```python
from build123d import *

# Parameters (mm, degrees)
EXTRUDE_1_DEPTH     = 30
CHAMFER_1_SIZE      = 5
SKETCH_2_R          = 4
CUT_EXTRUDE_2_DEPTH = 58.295890515
SKETCH_3_R          = 4
CUT_EXTRUDE_3_DEPTH = 61.952262634


with BuildPart() as part:
    # Эскиз1 → Вытянуть1 (new body)
    with BuildSketch(Plane.XY):
        Polygon((15, 7.896395833), (35, 7.896395833), (44.894389845, -8.278473804), (44.894389845, -28.278473804), (35, -28.278473804), (35, -8.278473804), (15, -8.278473804), (15, -28.278473804), (5.105610155, -28.278473804), (5.105610155, -8.278473804), align=None)
    extrude(amount=EXTRUDE_1_DEPTH)

    # Фаска1
    chamfer_1_edges = [part.edges().sort_by_distance(p)[0] for p in [
        (10.052805078, -28.278473804, 0),
        (39.947194922, -28.278473804, 0),
        (10.052805078, -28.278473804, 30),
        (39.947194922, -28.278473804, 30),
    ]]
    chamfer(chamfer_1_edges, length=CHAMFER_1_SIZE)

    # Эскиз2 → Вытянуть2 (cut, through all)
    with BuildSketch(Plane.ZY.offset(-5.105610155)):
        with Locations((15, -18.278473804)):
            Circle(SKETCH_2_R)
    extrude(amount=-CUT_EXTRUDE_2_DEPTH, mode=Mode.SUBTRACT)

    # Эскиз3 → Вытянуть3 (cut, through all)
    with BuildSketch(Plane.XY.offset(30)):
        with Locations((25, -0.278473804)):
            Circle(SKETCH_3_R)
    extrude(amount=-CUT_EXTRUDE_3_DEPTH, mode=Mode.SUBTRACT)


solid = part.part
```
Check sheet for the modelled part. Datum: model origin and axes. Units: mm. A direction names the side the tool comes from. Round coordinates to 2 decimals unless told otherwise and drop trailing zeros. Loops run counter-clockwise (first coordinate to the right, second up) from the corner with the lowest first, then second, coordinate; pieces in that order, holes last. Notation, with made-up numbers: M 56,75 L 106,75 A32 ccw 106,107 Z; hole C 4.25,-40 d9. An arc over 180 degrees is marked long. Answer as a JSON object with one key per item and string values.
1. Section check D-D (z = 21). Record the boundary of the cut face in (x, y), plus the area to 3 significant figures.
Reply:
{"outline": "M 5.11,-28.28 L 15,-28.28 L 15,-8.28 L 35,-8.28 L 35,-28.28 L 44.89,-28.28 L 44.89,-8.28 L 35,7.9 L 15,7.9 L 5.11,-8.28 Z; hole C 25,-0.28 d8", "area": "829 mm²"}
2. Mould release check, pull along Z, two halves, no side actions. Record for faces 1 (the cylindrical face through (39.878, -18.103, 11.004)), 2 (the flat face through (40.02, -25.74, 2.46)), 3 (the flat face through (40, -28.278, 15)): pulls with the +Z half, pulls with the -Z half, needs draft (parallel to the pull), parting line crosses it, or undercut.
Reply:
{"face 1": "undercut", "face 2": "pulls with the -Z half", "face 3": "needs draft"}
3. Access from +Z, -Z, +X, -X, +Y, -Y to the whole of each face (thin tool, end or side, straight path). Record for faces 4 (the flat face through (10.12, -25.74, 27.54)), 5 (the flat face through (35, -16, 11)).
Reply:
{"face 4": "+Z, +X, -X, -Y", "face 5": "+Z, -Z, -Y"}
4. Section check C-C (x = 25). Record the boundary of the cut face in (y, z), plus the area to 3 significant figures.
Reply:
{"outline": "M -8.28,0 L -4.28,0 L -4.28,30 L -8.28,30 Z; M 3.72,0 L 7.9,0 L 7.9,30 L 3.72,30 Z", "area": "245 mm²"}
5. Section check B-B (y = -10.5). Record the boundary of the cut face in (x, z), plus the area to 3 significant figures.
Reply:
{"outline": "M 5.11,0 L 15,0 L 15,30 L 5.11,30 Z; M 35,0 L 44.89,0 L 44.89,30 L 35,30 Z", "area": "594 mm²"}
6. Gauge pin test, flat ends, axial feed: P1, Ø3, axis at y = -0.5, z = 19.5, coming from the -X side; P2, Ø10, axis at x = 23.5, z = 16.5, coming from the -Y side; P3, Ø6, axis at x = 10, z = 22.5, coming from the +Y side. Record the tip position at first contact, or that the pin passes through.
Reply:
{"P1": "stops at x = 8.95", "P2": "stops at y = -8.28", "P3": "stops at y = 4.63"}
7. Scan lines: line 1 (X direction, y = -23.5, z = 28.5); line 2 (Y direction, x = 30.5, z = 6.25); line 3 (Y direction, x = 23.5, z = 22). Record each from-to range of solid material in increasing order.
Reply:
{"line 1": "x = 5.11 to 15, 35 to 44.89", "line 2": "y = -8.28 to 7.9", "line 3": "y = -8.28 to -3.99, 3.43 to 7.9"}
8. Section check A-A (z = 15). Record the boundary of the cut face in (x, y).
Reply:
{"outline": "M 5.11,-28.28 L 15,-28.28 L 15,-22.28 L 5.11,-22.28 Z; M 5.11,-14.28 L 15,-14.28 L 15,-8.28 L 35,-8.28 L 35,-14.28 L 44.89,-14.28 L 44.89,-8.28 L 35,7.9 L 15,7.9 L 5.11,-8.28 Z; M 35,-28.28 L 44.89,-28.28 L 44.89,-22.28 L 35,-22.28 Z; hole C 25,-0.28 d8"}
